Autodesk Inventor part; units mm, degrees
ref_plane "YZ Plane" through (0, 0, 0) normal (1, 0, 0) x (0, 1, 0)
ref_plane "XZ Plane" through (0, 0, 0) normal (0, 1, 0) x (-1, 0, 0)
ref_plane "XY Plane" through (0, 0, 0) normal (0, 0, 1) x (1, 0, 0)
sketch "Эскиз1" plane through (0, 0, 0) normal (0, 1, 0) x (-1, 0, 0)
  line L0 (-11.5, 6.2) -> (11.5, 6.2)
  line L1 (11.5, 6.2) -> (11.5, -6.2)
  line L2 (11.5, -6.2) -> (-11.5, -6.2)
  line L3 (-11.5, -6.2) -> (-11.5, 6.2)
  line L4 (-11.5, 6.2) -> (11.5, -6.2) construction
  line L5 (11.5, 6.2) -> (-11.5, -6.2) construction
  point P0 (0, 0)
  dimension "d0" = 12.4
  dimension "d1" = 23
extrude "Выдавливание1" add sketch "Эскиз1" along normal blind 10.5
sketch "Эскиз2" plane through (0, 0, 0) normal (0, -1, 0) x (1, 0, 0)
  line L0 (11.5, 6.2) -> (-11.5, 6.2)
  line L1 (-11.5, 6.2) -> (-11.5, -6.2)
  line L2 (-11.5, -6.2) -> (11.5, -6.2)
  line L3 (11.5, -6.2) -> (11.5, 6.2)
  line L4 (-10.5, 5.2) -> (10.5, 5.2)
  line L5 (10.5, 5.2) -> (10.5, -5.2)
  line L6 (10.5, -5.2) -> (-10.5, -5.2)
  line L7 (-10.5, -5.2) -> (-10.5, 5.2)
  point P0 (0, 0)
  dimension "d66" = 1
extrude "Выдавливание2" cut sketch "Эскиз2" against normal blind 9.5 contours L4 L5 L6 L7
chamfer "Фаска1" distance 1.5 angle 45 4 edges at (-10.5, 4.75, 5.2) (10.5, 4.75, 5.2) (10.5, 4.75, -5.2) (-10.5, 4.75, -5.2)
sketch "Эскиз3" plane through (0, 9.5, 0) normal (0, -1, 0) x (1, 0, 0)
  line L0 (9, -5.2) -> (-9, -5.2)
  line L1 (-4, -5.2) -> (-2.5, -3.7)
  line L2 (-2.5, -3.7) -> (-2.5, 3.7)
  line L3 (-2.5, 3.7) -> (-4, 5.2)
  line L4 (-9, 5.2) -> (9, 5.2)
  line L5 (-16.1, 0) -> (16.1, 0)
  line L6 (-10.5, -3.7) -> (-10.5, 3.7)
  line L7 (-2.5858, 5.2) -> (-1.5, 4.1142)
  line L8 (-1.5, 4.1142) -> (-1.5, -4.1142)
  line L9 (-1.5, -4.1142) -> (-2.5858, -5.2)
  point P0 (0, 0)
  dimension "d9" = 1.5
  dimension "d10" = 8
  dimension "d11" = 1
  dimension "d12" = 1
extrude "Выдавливание3" add sketch "Эскиз3" along normal blind 4
sketch "Эскиз4" plane through (0, 5.5, 0) normal (0, -1, 0) x (1, 0, 0)
  line L0 (-2.5, 3.7) -> (-2.5, -3.7)
  line L1 (-1.5, -4.1142) -> (-1.5, 4.1142)
  line L2 (-2.5, 3.7) -> (-1.5, 3.7)
  line L3 (-1.5, 3.7) -> (-1.5, -3.7)
  line L4 (-1.5, -3.7) -> (-2.5, -3.7)
  line L5 (-2.5, -3.7) -> (-2.5, 3.7)
  point P0 (0, 0)
extrude "Выдавливание4" add sketch "Эскиз4" along normal blind 1
sketch "Эскиз5" plane through (0, 9.5, 0) normal (0, -1, 0) x (1, 0, 0)
  line L0 (-10.5, -3.7) -> (-10.5, 3.7)
  line L1 (-2.5, -3.7) -> (-2.5, 3.7)
  line L2 (-9, 5.2) -> (9, 5.2)
  line L3 (9, -5.2) -> (-9, -5.2)
  line L4 (-2.5, 3.7) -> (-2.5, -3.7)
  point P0 (0, 0)
  point P1 (-6.5, 0)
  point P2 (-2.5, 0)
  dimension "d64" = 8
  dimension "d65" = 4
hole "Отверстие1" at (-6.5, 9.5, 0) direction (0, 1, 0) diameter 4.1 depth 8 tip angle 118
sketch "Эскиз6" plane through (0, 9.5, 0) normal (0, -1, 0) x (1, 0, 0)
  circle A0 centre (5.5, 0) radius 5
  line L0 (10.5, 3.7) -> (10.5, -3.7)
  line L1 (-16.1, 0) -> (16.1, 0)
  line L2 (10.5, 3.7) -> (10.5, -3.7)
  circle A1 centre (5.5, 0) radius 6
  point P0 (0, 0)
  dimension "d24" = 10
  dimension "d25" = 1
extrude "Выдавливание5" add sketch "Эскиз6" along normal blind 4 contours L0 A1 L1 A0 | A0 L1 A1 L0 | L1 A1 L0 | L0 A1 L1
sketch "Эскиз7" plane through (5.5, 9.5, 0) normal (0, -1, 0) x (1, 0, 0)
  circle A0 centre (0, 0) radius 5
  circle A1 centre (0, 0) radius 4.5
  point P0 (-5.5, 0)
  dimension "d28" = 9
extrude "Выдавливание6" cut sketch "Эскиз7" against normal blind 5 contours A1
sketch "Эскиз8" plane through (5.5, 9.5, 0) normal (0, -1, 0) x (1, 0, 0)
  circle A0 centre (0, 0) radius 4.5
  circle A1 centre (0, 0) radius 5
  point P0 (-5.5, 0)
extrude "Выдавливание7" add sketch "Эскиз8" along normal blind 2
sketch "Эскиз9" plane through (0, 10.5, 0) normal (0, 1, 0) x (1, 0, 0)
  circle A0 centre (5.5, 0) radius 4.5
  circle A1 centre (5.5, 0) radius 5
  point P0 (0, 0)
  dimension "d33" = 10
extrude "Выдавливание8" cut sketch "Эскиз9" against normal blind 1
sketch "Эскиз10" plane through (0, 5.5, 0) normal (0, -1, 0) x (1, 0, 0)
  line L0 (2.5067, 5.2) -> (8.4933, 5.2)
  line L1 (4.5, 5.2) -> (6.5, 5.2)
  line L2 (6.5, 5.2) -> (6.5, 3.2)
  line L3 (6.5, 3.2) -> (4.5, 3.2)
  line L4 (4.5, 3.2) -> (4.5, 5.2)
  line L5 (9, -5.2) -> (-9, -5.2)
  line L6 (4.5, -5.2) -> (6.5, -5.2)
  line L7 (6.5, -5.2) -> (6.5, -3.2)
  line L8 (6.5, -3.2) -> (4.5, -3.2)
  line L9 (4.5, -3.2) -> (4.5, -5.2)
  line L10 (-16.1, 0) -> (16.1, 0)
  circle A0 centre (5.5, 0) radius 4.5
  point P0 (0, 0)
  point P1 (5.5, 3.2)
  dimension "d36" = 2
  dimension "d37" = 2
extrude "Выдавливание9" add sketch "Эскиз10" against normal blind 0.5 contours L0 L2 A0 L4 | A0 L2 L3 L4 | A0 L7 L5 L9 | L9 L8 L7 A0
sketch "Эскиз11" plane through (0, 9.5, 0) normal (0, -1, 0) x (1, 0, 0)
  circle A0 centre (-0.5, 0) radius 1
  line L0 (-11.5, 6.2) -> (-11.5, -6.2)
  point P0 (0, 0)
  dimension "d40" = 11
  dimension "d41" = 2
extrude "Выдавливание10" add sketch "Эскиз11" along normal blind 2
sketch "Эскиз12" plane through (0, 10.5, 0) normal (0, 1, 0) x (1, 0, 0)
  arc A0 (-1.5, 0) -> (-0.4167, -0.9965) centre (-0.5, 0) ccw
  line L0 (-11.5, 6.2) -> (-11.5, -6.2)
  circle A1 centre (-6.428, 0) radius 2.05
  point P0 (0, 0)
  point P1 (-1.5, -0.866)
  dimension "d63" = 11
hole "Отверстие2" at (-0.5, 10.5, 0) direction (0, -1, 0) diameter 1.2 depth 2
sketch "Эскиз13" plane through (0, 0, 0) normal (0, -1, 0) x (1, 0, 0)
  line L0 (-10, -4.5) -> (10, -4.5)
  line L1 (10, -4.5) -> (10, 4.5)
  line L2 (10, 4.5) -> (-10, 4.5)
  line L3 (-10, 4.5) -> (-10, -4.5)
  line L4 (-10, -4.5) -> (10, 4.5) construction
  line L5 (10, -4.5) -> (-10, 4.5) construction
  point P0 (0, 0)
  dimension "d51" = 9
  dimension "d52" = 20
hole "Отверстие3" at (10, 0, 4.5) at (10, 0, -4.5) at (-10, 0, 4.5) at (-10, 0, -4.5) direction (0, 1, 0) diameter 1.4 depth 12 tip angle 118
sketch "Эскиз14" plane through (0, 10.5, 0) normal (0, 1, 0) x (1, 0, 0)
  circle A0 centre (10, 4.5) radius 0.7
  circle A1 centre (10, -4.5) radius 0.7
  circle A2 centre (-10, -4.5) radius 0.7
  circle A3 centre (-10, 4.5) radius 0.7
  circle A4 centre (10, 4.5) radius 0.9
  circle A5 centre (-10, 4.5) radius 0.9
  circle A6 centre (-10, -4.5) radius 0.9
  circle A7 centre (10, -4.5) radius 0.9
  circle A8 centre (-0.5, 0) radius 0.6
  circle A9 centre (-0.5, 0) radius 0.9
  point P0 (0, 0)
  dimension "d60" = 1.8
extrude "Выдавливание11" add sketch "Эскиз14" along normal blind 0.4
properties part number "основание крпуса редуктора" material "Пластик ПК/АБС"
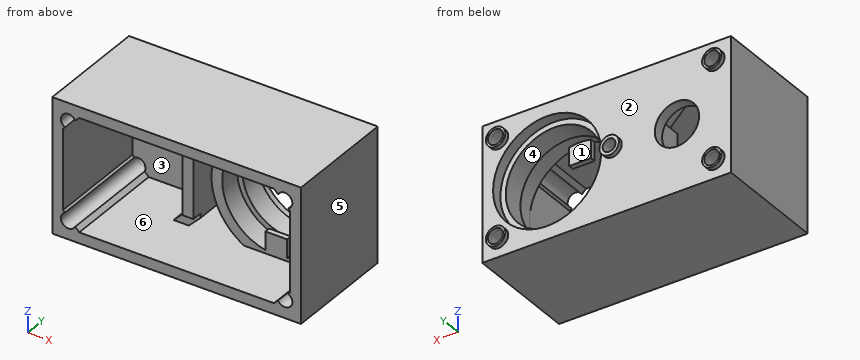
Could you check a few things on this model? Use its own coordinates, in mm. Face numbers are marked on the shaded views. A direction names the side the tool comes from. Coordinates: 2 decimals unless noted, no trailing zeros. Order: outer loops, then holes, each group sorted by start corner. A loop starts at its lowest first (then second) coordinate and runs counter-clockwise, first axis right, second up.
Q1. Suppose I cut it at C-C on y = 2. Please give me the cut outline in (x, z).
Q2. Suppose I cut it at B-B on x = -6.5. Please give me the cut outline in (y, z), and give its area (3 significant figures).
Q3. Will these pins go through, and if not, where does the flat tip stop? pin 1 (1 mm diameter, centred on x = -1.5, z = 4.5, fed in from +Y); pin 2 (5.5 mm diameter, centred on x = -6.5, z = 0, fed in from -Y); pin 3 (1 mm diameter, centred on x = -0.5, z = 0, fed in from +Y).
Q4. Which directions (+Z, -Z, +X, -X, +Y, -Y) give clear straight access to the entire face, cutting with the end or side of a thin tool? Please do the marked faces 5 and 6.
Q5. Suppose I cut it at A-A on x = -10. Please give me the cut outline in (y, z).
Q6. Thinking about a two-plate mould opening in Y: for the marked faces 1, 2, 3 and 4, which applies, released by +Y, released by -Y, zero draft, split by the parting line, or undercut?
Q7. Please list where these lines run through material, in increasing order: L1, parallel to Z at x = -10, y = 10.8; L2, parallel to Z at x = -10, y = 5; L3, parallel to X at y = 3.25, z = -0.5.
Q8. Suppose I cut it at D-D on z = -1.75. Give the number of separate pieces and of enclosed holes in the cut face, and give its area (3 significant figures).
Answer:
1. outline: (-11.5, -6.2) - (11.5, -6.2) - (11.5, 6.2) - (-11.5, 6.2) - close; hole (-10.5, -3.7) - (-10.32, -3.88) arc R0.7 ccw (long way) to (-9.38, -4.82) - (-9, -5.2) - (9, -5.2) - (9.38, -4.82) arc R0.7 ccw (long way) to (10.32, -3.88) - (10.5, -3.7) - (10.5, 3.7) - (10.32, 3.88) arc R0.7 ccw (long way) to (9.38, 4.82) - (9, 5.2) - (-9, 5.2) - (-9.38, 4.82) arc R0.7 ccw (long way) to (-10.32, 3.88) - (-10.5, 3.7) - close
2. outline: (0, -6.2) - (10.5, -6.2) - (10.5, -2.05) - (9.5, -2.05) - (9.5, -5.2) - (0, -5.2) - close; (0, 5.2) - (9.5, 5.2) - (9.5, 2.05) - (10.5, 2.05) - (10.5, 6.2) - (0, 6.2) - close
2. area: 27.3 mm2
3. pin 1: stops at y = 10.5
3. pin 2: stops at y = 9.5
3. pin 3: stops at y = 8.5
4. face 5: +Z, -Z, +X, +Y, -Y
4. face 6: -Y
5. outline: (0, -6.2) - (10.5, -6.2) - (10.5, -5.4) - (10.9, -5.4) - (10.9, -5.2) - (0, -5.2) - close; (0, 5.2) - (10.9, 5.2) - (10.9, 5.4) - (10.5, 5.4) - (10.5, 6.2) - (0, 6.2) - close; (9.5, -3.8) - (10.9, -3.8) - (10.9, -3.6) - (10.5, -3.6) - (10.5, 3.6) - (10.9, 3.6) - (10.9, 3.8) - (9.5, 3.8) - close
6. face 1: undercut
6. face 2: released by +Y
6. face 3: released by -Y
6. face 4: zero draft
7. L1: z = -5.4 to -5.2, -3.8 to -3.6, 3.6 to 3.8, 5.2 to 5.4
7. L2: z = -6.2 to -5.2, 5.2 to 6.2
7. L3: x = -11.5 to -10.5, 10.5 to 11.5
8. separate pieces: 3
8. enclosed holes: 0
8. area: 43.1 mm2
